```python
from build123d import *

# Parameters (mm, degrees)
RUNROUTE_R          = 16.75
RUNEXTRUDE_DEPTH    = 63.4
OUTLETROUTE_R       = 13.4
OUTLETEXTRUDE_DEPTH = 66.75
TEESHELL_T          = -3.2
TEECHAMFER_SIZE     = 1


with BuildPart() as part:
    # RunRoute → RunExtrude (new body)
    with BuildSketch(Plane(origin=(0, 0, 0), x_dir=(0, 0, -1), z_dir=(1, 0, 0))):
        Circle(RUNROUTE_R)
    runextrude = extrude(amount=RUNEXTRUDE_DEPTH)

    # RunExtrudeMirror: RunExtrude across plane
    add(runextrude.mirror(Plane(origin=(0, 0, 0), x_dir=(0, 0, 1), z_dir=(1, 0, 0))))

    # OutletRoute → OutletExtrude (add)
    with BuildSketch(Plane(origin=(0, 0, 0), x_dir=(1, 0, 0), z_dir=(0, 1, 0))):
        with Locations(Location((0, 0, 0), (0, 0, 90))):
            Circle(OUTLETROUTE_R)
    extrude(amount=OUTLETEXTRUDE_DEPTH)

    # TeeShell
    teeshell_openings = [part.faces().sort_by_distance(p)[0] for p in [
        (63.4, 0, 0),
        (0, 66.75, 0),
        (-63.4, 0, 0),
    ]]
    offset(amount=TEESHELL_T, openings=teeshell_openings, kind=Kind.INTERSECTION)

    # TeeChamfer
    teechamfer_edges = [part.edges().sort_by_distance(p)[0] for p in [
        (63.4, 0, 16.75),
        (-63.4, 0, 16.75),
        (0, 66.75, 13.4),
    ]]
    chamfer(teechamfer_edges, length=TEECHAMFER_SIZE)


solid = part.part
```
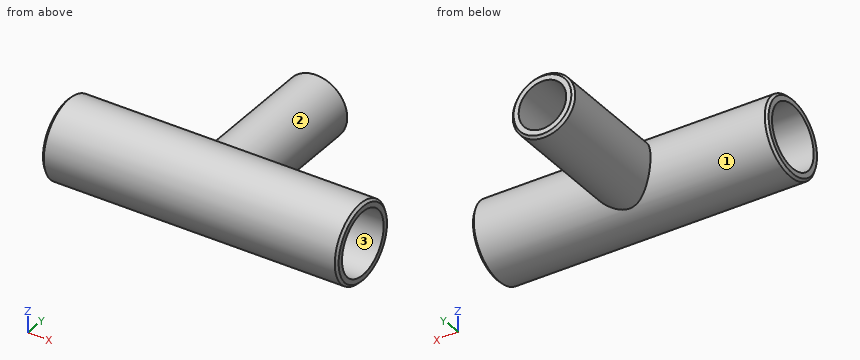
Read the model definition and answer for the solid it produces. Units are mm, in the model's axes. Face numbers are marked on the shaded views. Coordinates: 2 decimals unless noted, no trailing zeros. Loops run counter-clockwise (first coordinate to the right, second up) from the corner with the lowest first, then second, coordinate; pieces in that order, holes last. Notation, with made-up numbers: (63, 65) -> (76, 65) arc R25 ccw to (76, 87) -> close; hole circle Ø3 at (-32, 31.25). An arc over 180 degrees is marked (long way). Return JSON: item names as keys, results as strings.
Item 1: Find section B-B (z = 0). Determine the outline of the cut face in (x, y).
Answers:
{"outline": "(-63.4, -15.75) -> (-62.4, -16.75) -> (62.4, -16.75) -> (63.4, -15.75) -> (63.4, -13.55) -> (-63.4, -13.55) -> close; (-63.4, 13.55) -> (-10.2, 13.55) -> (-10.2, 66.75) -> (-12.4, 66.75) -> (-13.4, 65.75) -> (-13.4, 16.75) -> (-62.4, 16.75) -> (-63.4, 15.75) -> close; (10.2, 13.55) -> (63.4, 13.55) -> (63.4, 15.75) -> (62.4, 16.75) -> (13.4, 16.75) -> (13.4, 65.75) -> (12.4, 66.75) -> (10.2, 66.75) -> close"}
Item 2: Find section C-C (x = -55.5). Determine the outline of the cut face in (y, z).
Answers:
{"outline": "circle Ø33.5 at (0, 0); hole circle Ø27.1 at (0, 0)"}
Item 3: Flat-ended cylindrical pins translate along their axes: P1, Ø10, axis at y = 51, z = 7.5, coming from the +X side; P2, Ø12, axis at y = 56.5, z = -3, coming from the -X side; P3, Ø1, axis at x = 44.5, y = 9.5, coming from the -Z side. Find the tip coordinate at first contact, or state that the pin passes through.
Answers:
{"P1": "stops at x = 13.16", "P2": "stops at x = -13.4", "P3": "stops at z = -14.13"}
Item 4: For a pull along Y with two mould halves and no side action, classify the marked faces 1, 2 and 3 as +Y half, -Y half, draft (parallel to the pull), parting line (faces both ways), or undercut.
Answers:
{"face 1": "parting line", "face 2": "draft", "face 3": "undercut"}
Item 5: Find the intervals of material crossed by probe 1 along X at (y, z) = (53, 0); probe 2 along Z at (x, y) = (1, 61); probe 3 along Y at (x, z) = (-28, 0), in increasing order.
Answers:
{"probe 1": "x = -13.4 to -10.2, 10.2 to 13.4", "probe 2": "z = -13.36 to -10.15, 10.15 to 13.36", "probe 3": "y = -16.75 to -13.55, 13.55 to 16.75"}
Item 6: Find section A-A (y = 0). Determine the outline of the cut face in (x, z), plus the area to 3 significant figures.
Answers:
{"outline": "(-63.4, -15.75) -> (-62.4, -16.75) -> (62.4, -16.75) -> (63.4, -15.75) -> (63.4, -13.55) -> (-63.4, -13.55) -> close; (-63.4, 13.55) -> (63.4, 13.55) -> (63.4, 15.75) -> (62.4, 16.75) -> (-62.4, 16.75) -> (-63.4, 15.75) -> close", "area": "810 mm2"}
Item 7: Find section D-D (x = 0). Determine the outline of the cut face in (y, z), plus the area to 3 significant figures.
Answers:
{"outline": "(8.92, -10.2) arc R13.55 cw (long way) to (8.92, 10.2) -> (66.75, 10.2) -> (66.75, 12.4) -> (65.75, 13.4) -> (10.05, 13.4) arc R16.75 ccw (long way) to (10.05, -13.4) -> (65.75, -13.4) -> (66.75, -12.4) -> (66.75, -10.2) -> close", "area": "583 mm2"}
